from build123d import *

# Parameters (mm, degrees)
SKETCH_1_W      = 40
SKETCH_1_H      = 39
SKETCH_1_R      = 1.5
SKETCH_1_H_2    = 2
EXTRUDE_2_DEPTH = 2
EXTRUDE_3_DEPTH = 2
FILLET_1_R      = 1
FILLET_2_R      = 3


with BuildPart() as part:
    # 草图1 → 凸台-拉伸2 (new body)
    with BuildSketch(Plane.XY):
        with Locations((0, -1)):
            Rectangle(SKETCH_1_W, SKETCH_1_H)
        with Locations((-15, -12.5)):
            Circle(SKETCH_1_R, mode=Mode.SUBTRACT)
        with Locations((15, -12.5)):
            Circle(SKETCH_1_R, mode=Mode.SUBTRACT)
        with Locations((-15, 11.5)):
            Circle(SKETCH_1_R, mode=Mode.SUBTRACT)
        with Locations((15, 11.5)):
            Circle(SKETCH_1_R, mode=Mode.SUBTRACT)
        with Locations((0, 19.5)):
            Rectangle(SKETCH_1_W, SKETCH_1_H_2)
    extrude(amount=EXTRUDE_2_DEPTH)

    # 草图2 → 凸台-拉伸3 (add)
    with BuildSketch(Plane(origin=(0, 18.5, 0), x_dir=(1, 0, 0), z_dir=(0, 1, 0))):
        with BuildLine():
            ThreePointArc((20, 24.5), (0, 44.5), (-20, 24.5))
            Line((-20, 24.5), (-17, 24.5))
            ThreePointArc((-17, 24.5), (-15.5, 26), (-14, 24.5))
            Line((-14, 24.5), (-6.5, 24.5))
            Line((-6.5, 24.5), (-6.5, 31.5))
            ThreePointArc((-6.5, 31.5), (0, 38), (6.5, 31.5))
            Line((6.5, 31.5), (6.5, 24.5))
            Line((6.5, 24.5), (13.998241038, 24.5))
            ThreePointArc((13.998241038, 24.5), (15.5, 26.001758962), (17.001758962, 24.5))
            Line((17.001758962, 24.5), (20, 24.5))
        make_face()
        with BuildLine():
            Line((-17, 24.5), (-20, 24.5))
            ThreePointArc((-20, 24.5), (0, 4.5), (20, 24.5))
            Line((20, 24.5), (17.001758962, 24.5))
            ThreePointArc((17.001758962, 24.5), (15.5, 22.998241038), (13.998241038, 24.5))
            Line((13.998241038, 24.5), (6.5, 24.5))
            Line((6.5, 24.5), (6.5, 17.5))
            ThreePointArc((6.5, 17.5), (0, 11), (-6.5, 17.5))
            Line((-6.5, 17.5), (-6.5, 24.5))
            Line((-6.5, 24.5), (-14, 24.5))
            ThreePointArc((-14, 24.5), (-15.5, 23), (-17, 24.5))
        make_face()
        with BuildLine():
            Line((-20, 24.5), (-20, -2))
            Line((-20, -2), (20, -2))
            Line((20, -2), (20, 24.5))
            ThreePointArc((20, 24.5), (0, 4.5), (-20, 24.5))
        make_face()
    extrude(amount=EXTRUDE_3_DEPTH)

    # 圆角1
    fillet_1_edges = [part.edges().sort_by_distance(p)[0] for p in [
        (0, 18.5, 0),
        (0, 20.5, 2),
    ]]
    fillet(fillet_1_edges, radius=FILLET_1_R)

    # 圆角2
    fillet_2_edges = [part.edges().sort_by_distance(p)[0] for p in [
        (20, -20.5, 1),
        (-20, -20.5, 1),
    ]]
    fillet(fillet_2_edges, radius=FILLET_2_R)


solid = part.part
Design review of the part built by this model. Coordinates are the model's own, in mm. A direction names the side the tool comes from. Coordinates: 2 decimals unless noted, no trailing zeros. Order: outer loops, then holes, each group sorted by start corner. A loop starts at its lowest first (then second) coordinate and runs counter-clockwise, first axis right, second up. Notation, with made-up numbers: M 24,74.5 L 35,74.5 A30 ccw 35,106.5 Z; hole C -25,-10.5 d6. An arc over 180 degrees is marked long. Use a Markdown table: item, result.
(1) Wall thickness on probe 1 along Y at (x, z) = (-15, 1.15); probe 2 along Y at (x, z) = (-15, 1.55); probe 3 along Z at (x, y) = (0.5, 11.5): over which ranges is each line inside the solid? List them lowest first.
Worked answers:
| item | result |
|---|---|
| probe 1 | y = -20.5 to -14, -11 to 10, 13 to 20.49 |
| probe 2 | y = -20.5 to -14, -11 to 10, 13 to 20.34 |
| probe 3 | z = 0 to 2 |
(2) Draft analysis for pull direction X (two halves, no side actions). For faces 4 (the cylindrical face through (19.14, -19.6, 1.01)), 5 (the flat face through (0, 0, 2)), 6 (the cylindrical face through (-16.61, 19.49, -23.49)), state which applies: released by +X, released by -X, zero draft, split by the parting line, or undercut.
Worked answers:
| item | result |
|---|---|
| face 4 | released by +X |
| face 5 | zero draft |
| face 6 | undercut |
(3) Add section D-D (x = -15). Give the boundary of the cut face in (y, z).
Worked answers:
| item | result |
|---|---|
| outline | M -20.5,0 L -14,0 L -14,2 L -20.5,2 Z; M -11,0 L 10,0 L 10,2 L -11,2 Z; M 13,0 L 17.5,0 A1 cw 18.5,-1 L 18.5,-23.09 L 20.5,-23.09 L 20.5,1 A1 ccw 19.5,2 L 13,2 Z; M 18.5,-37.73 L 20.5,-37.73 L 20.5,-25.91 L 18.5,-25.91 Z |
(4) Add section B-B (y = 11.5). Give the boundary of the cut face in (x, z), then the cut area to 3 significant figures.
Worked answers:
| item | result |
|---|---|
| outline | M -20,0 L -16.5,0 L -16.5,2 L -20,2 Z; M -13.5,0 L 13.5,0 L 13.5,2 L -13.5,2 Z; M 16.5,0 L 20,0 L 20,2 L 16.5,2 Z |
| area | 68.0 mm2 |
(5) Add section A-A (x = 0). Give the boundary of the cut face in (y, z).
Worked answers:
| item | result |
|---|---|
| outline | M -20.5,0 L 17.5,0 A1 cw 18.5,-1 L 18.5,-11 L 20.5,-11 L 20.5,1 A1 ccw 19.5,2 L -20.5,2 Z; M 18.5,-44.5 L 20.5,-44.5 L 20.5,-38 L 18.5,-38 Z |
(6) For faces 1 (the flat face through (-20, 7, 0.5)), 2 (the flat face through (0, -1, 0)), 3 (the flat face through (6.5, 19, -25)), list the 3-axis set-ups (+Z, -Z, +X, -X, +Y, -Y) from which the entire face can be reached by the end or side of a thin tool; tool diameter is ignored.
Worked answers:
| item | result |
|---|---|
| face 1 | +Z, -Z, -X, +Y, -Y |
| face 2 | -Z, +X, -X, -Y |
| face 3 | +Y, -Y |
(7) Add section C-C (z = -14). Give the boundary of the cut face in (x, y), then the cut area to 3 significant figures.
Worked answers:
| item | result |
|---|---|
| outline | M -20,18.5 L -5.48,18.5 L -5.48,20.5 L -20,20.5 Z; M 5.48,18.5 L 20,18.5 L 20,20.5 L 5.48,20.5 Z |
| area | 58.1 mm2 |
(8) For P1, Ø1, axis at x = -2.5, y = 4, coming from the -Z side; P2, Ø3, axis at x = -14.5, z = -21, coming from the -Y side, all flat-tipped, find the tip position at first contact; note any pin that passes through.
Worked answers:
| item | result |
|---|---|
| P1 | stops at z = 0 |
| P2 | stops at y = 18.5 |
